```python
from build123d import *

# Parameters (mm, degrees)
SKETCH1_R           = 2
SKETCH1_W           = 12.7
SKETCH1_H           = 50.8
BOSS_EXTRUDE3_DEPTH = 6.35
SKETCH2_R           = 1.5
CUT_EXTRUDE2_DEPTH  = 10


with BuildPart() as part:
    # Sketch1 → Boss-Extrude3 (new body)
    with BuildSketch(Plane(origin=(0, 0, 0), x_dir=(1, 0, 0), z_dir=(0, 1, 0))):
        with BuildLine():
            ThreePointArc((34.194833578, -66.63583839), (33.11372382, -66.748004461), (32.240681933, -66.10056535))
            ThreePointArc((32.240681933, -66.10056535), (0, -48.302004425), (-32.240681933, -66.10056535))
            ThreePointArc((-32.240681933, -66.10056535), (-33.11372382, -66.748004461), (-34.194833578, -66.63583839))
            ThreePointArc((-34.194833578, -66.63583839), (0, 74.897407173), (34.194833578, -66.63583839))
        make_face()
        with Locations((0, 53.061187965)):
            Circle(SKETCH1_R, mode=Mode.SUBTRACT)
        with Locations((18.178952795, 24.310551096)):
            Circle(SKETCH1_R, mode=Mode.SUBTRACT)
        with Locations((46.663733983, 40.081231883)):
            Circle(SKETCH1_R, mode=Mode.SUBTRACT)
        with Locations((46.663733983, -40.081231883)):
            Circle(SKETCH1_R, mode=Mode.SUBTRACT)
        with Locations((-46.663733983, -40.081231883)):
            Circle(SKETCH1_R, mode=Mode.SUBTRACT)
        with Locations((-18.178952795, 24.310551096)):
            Circle(SKETCH1_R, mode=Mode.SUBTRACT)
        with Locations((-46.663733983, 40.081231883)):
            Circle(SKETCH1_R, mode=Mode.SUBTRACT)
        with Locations((61.164123727, 0)):
            Rectangle(SKETCH1_W, SKETCH1_H, mode=Mode.SUBTRACT)
        with Locations((-61.164123727, 0)):
            Rectangle(SKETCH1_W, SKETCH1_H, mode=Mode.SUBTRACT)
        with BuildLine():
            ThreePointArc((-5.853899988, 60.78531778), (0.003726822, 57.376699875), (5.857575472, 60.791802193))
            ThreePointArc((5.857575472, 60.791802193), (10.16, 64.107698843), (5.857575472, 67.423595493))
            ThreePointArc((5.857575472, 67.423595493), (0.003726822, 70.838697812), (-5.853899988, 67.430079907))
            ThreePointArc((-5.853899988, 67.430079907), (-10.167207264, 64.107698843), (-5.853899988, 60.78531778))
        make_face(mode=Mode.SUBTRACT)
    extrude(amount=BOSS_EXTRUDE3_DEPTH)

    # Sketch2 → Cut-Extrude2 (cut)
    with BuildSketch(Plane(origin=(0, 0, 0), x_dir=(1, 0, 0), z_dir=(0, 1, 0))):
        with Locations((-47.745737366, 11.205)):
            Circle(SKETCH2_R)
        with Locations((-47.745737366, -11.205)):
            Circle(SKETCH2_R)
        with Locations((-15.945737366, 11.205)):
            Circle(SKETCH2_R)
        with Locations((-15.945737366, -11.205)):
            Circle(SKETCH2_R)
        with Locations((15.945737366, -11.205)):
            Circle(SKETCH2_R)
        with Locations((15.945737366, 11.205)):
            Circle(SKETCH2_R)
        with Locations((47.745737366, -11.205)):
            Circle(SKETCH2_R)
        with Locations((47.745737366, 11.205)):
            Circle(SKETCH2_R)
    extrude(amount=CUT_EXTRUDE2_DEPTH, mode=Mode.SUBTRACT)


solid = part.part
```
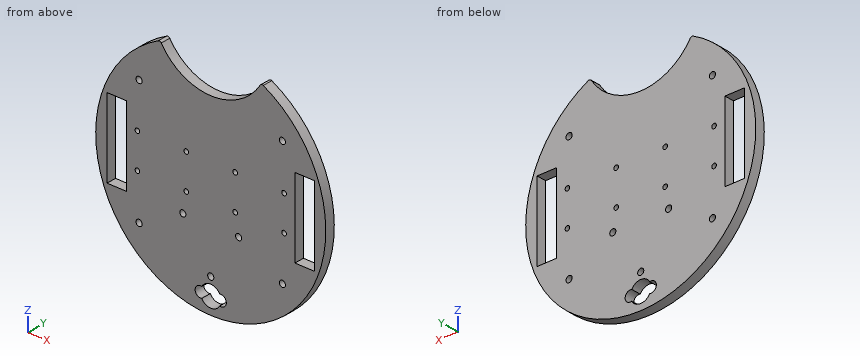
Verification items for the finished model (mm, model axes). Give positions to 0.01 mm unless a question says otherwise; leave off trailing zeros. Order: outer loops, then holes, each group sorted by start corner. A loop starts at its lowest first (then second) coordinate and runs counter-clockwise, first axis right, second up. Notation, with made-up numbers: M 38,68 L 80,68 A12 ccw 80,73 Z; hole C 82,-0.75 d9. An arc over 180 degrees is marked long. Answer in a Markdown table with one row per item. Add a question column.
Item 1: Section check B-B, the plane x = 0. Enter the section's corners in (y, z), and give its area (3 significant figures).
Item 2: Section check D-D, the plane x = -27.5. Enter the section's corners in (y, z), and give its area (3 significant figures).
Item 3: Section check A-A, the plane z = 0. Enter the section's corners in (x, y), and give its area (3 significant figures).
Item 4: Section check C-C, the plane y = 1. State how many separate pieces and enclosed holes the cut face has, and give its area (3 significant figures).
Item 5: Gauge pin test, flat ends, axial feed: pin 1 (2 mm diameter, centred on x = 14.5, y = 1.5, fed in from -Z); pin 2 (3 mm diameter, centred on x = -59.5, y = 2, fed in from -Z); pin 3 (1 mm diameter, centred on x = -43.5, y = 4, fed in from -Z). Record the tip position at first contact, or that the pin passes through.
Item 6: Scan lines: probe 1 along Z at (x, y) = (-15.5, 3.5); probe 2 along X at (y, z) = (2.25, -21.5); probe 3 along X at (y, z) = (1, -39.5). Record each from-to range of solid material in increasing order. Write a range as from..to.
Filled sheet:
| question | item | result |
|---|---|---|
| 1 | outline | M 0,-74.9 L 6.35,-74.9 L 6.35,-70.84 L 0,-70.84 Z; M 0,-57.38 L 6.35,-57.38 L 6.35,-55.06 L 0,-55.06 Z; M 0,-51.06 L 6.35,-51.06 L 6.35,48.3 L 0,48.3 Z |
| 1 | area | 671 mm^2 |
| 2 | outline | M 0,-69.67 L 6.35,-69.67 L 6.35,60.03 L 0,60.03 Z |
| 2 | area | 824 mm^2 |
| 3 | outline | M -74.9,0 L -67.51,0 L -67.51,6.35 L -74.9,6.35 Z; M -54.81,0 L 54.81,0 L 54.81,6.35 L -54.81,6.35 Z; M 67.51,0 L 74.9,0 L 74.9,6.35 L 67.51,6.35 Z |
| 3 | area | 790 mm^2 |
| 4 | separate pieces | 1 |
| 4 | enclosed holes | 18 |
| 4 | area | 14,800 mm^2 |
| 5 | pin 1 | stops at z = -73.67 |
| 5 | pin 2 | stops at z = -47.39 |
| 5 | pin 3 | stops at z = -61.32 |
| 6 | probe 1 | z = -73.28..-12.64, -9.77..9.77, 12.64..51.6 |
| 6 | probe 2 | x = -71.75..-67.51, -54.81..54.81, 67.51..71.75 |
| 6 | probe 3 | x = -63.63..-48.58, -44.75..44.75, 48.58..63.63 |
